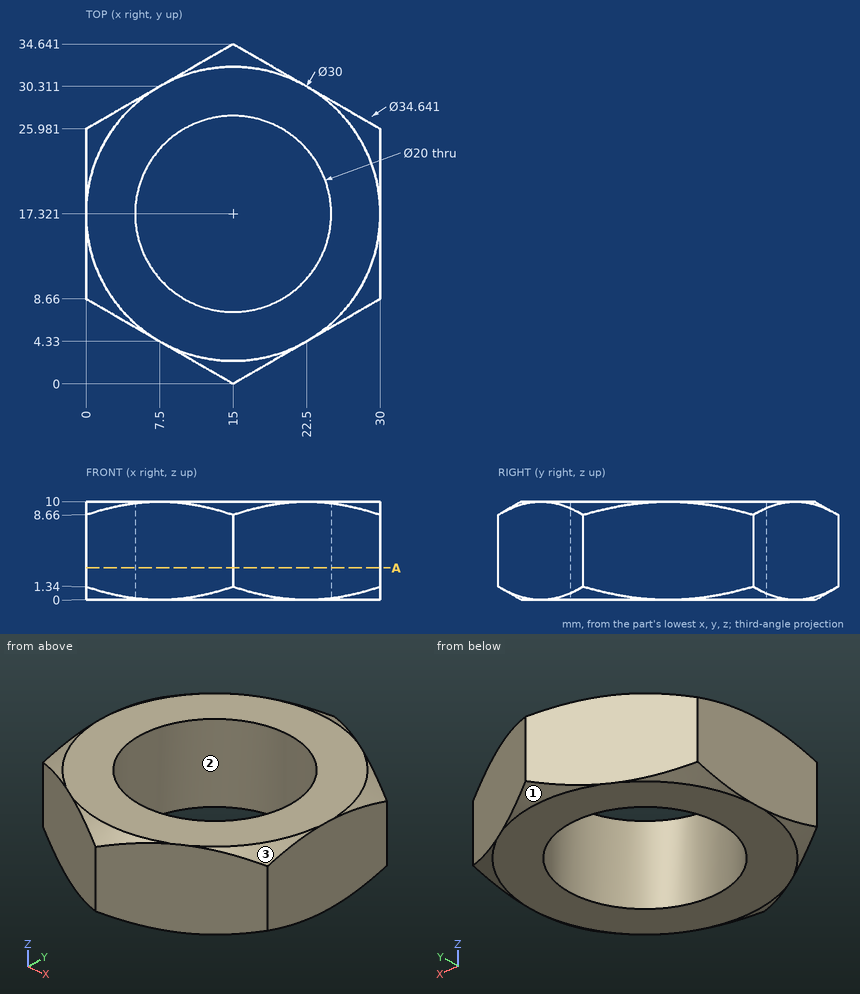
Design review of the part shown in the three views and the two pictorial views. Dimensions are in mm from the part's minimum x, y and z. Coordinates: 2 decimals unless noted, no trailing zeros. Order: outer loops, then holes, each group sorted by start corner. A loop starts at its lowest first (then second) coordinate and runs counter-clockwise, first axis right, second up. Notation, with made-up numbers: (52, 51.5) - (63, 51.5) arc R12 cw to (63, 67.5) - close; hole circle Ø8 at (38.5, 66.5). An arc over 180 degrees is marked (long way). One line per question, with ' | ' between items.
Q1. Consider section A-A, the plane z = 3.25. Give the boundary of the cut face in (x, y), then the cut area to 3 significant figures.
Answer key:
outline: (0, 8.66) - (15, 0) - (30, 8.66) - (30, 25.98) - (15, 34.64) - (0, 25.98) - close; hole circle Ø20 at (15, 17.32) | area: 465 mm2
Q2. The part is to be moulded in two halves that separate along X. For the marked faces 1, 2 and 3, say which applies: +X half, -X half, draft (parallel to the pull), parting line (faces both ways), or undercut.
Answer key:
face 1: parting line | face 2: undercut | face 3: +X half
Q3. Clearance check with flat-ended pins moving along their axes: pin 1 Ø3 at (y, z) = (3.5, 8.5) entering from +X; pin 2 Ø4 at (x, z) = (26, 5.5) entering from +Y (1 decimal). State where each tip first meets the part, or that it passes through.
Answer key:
pin 1: stops at x = 23.66 | pin 2: stops at y = 29.4
Q4. To check wall thickness, follow line 1 along Y through (x, z) = (15, 3); line 2 along X through (y, z) = (15, 3.5); line 3 along Y through (x, z) = (8, 5.75). State the ranges of each line that lie inside material, in increasing order.
Answer key:
line 1: y = 0 to 7.32, 27.32 to 34.64 | line 2: x = 0 to 5.27, 24.73 to 30 | line 3: y = 4.04 to 10.18, 24.46 to 30.6
